Could you check a few things on this model? Use its own coordinates, in mm. A direction names the side the tool comes from. Round coordinates to 2 decimals unless told otherwise and drop trailing zeros. Write each loop counter-clockwise with the first axis right and the second up, starting at its lowest first coordinate (ties: lowest second). Pieces come first, ordered by that corner, then holes.
```python
from build123d import *

# Parameters (mm, degrees)
F0_R     = 9.525
F1_DEPTH = 12.7


with BuildPart() as f1:
    # F0 (on Top) → F1 (new body, symmetric)
    with BuildSketch(Plane.XY):
        with BuildLine():
            ThreePointArc((0, 38.1), (9.715033, 36.840577), (18.787791, 33.145571))
            Line((18.787791, 33.145571), (0, 50.8))
            Line((0, 50.8), (0, 38.1))
        make_face()
        with BuildLine():
            ThreePointArc((-20.773422, 31.938612), (-10.838983, 36.525696), (-0.010502, 38.099999))
            Line((-0.010502, 38.099999), (-25.138711, 43.864812))
            Line((-25.138711, 43.864812), (-20.773422, 31.938612))
        make_face()
        with BuildLine():
            ThreePointArc((-34.823787, 15.45684), (-28.994389, 24.717107), (-20.773422, 31.938612))
            Line((-20.773422, 31.938612), (-44.983609, 23.077076))
            Line((-44.983609, 23.077076), (-34.823787, 15.45684))
        make_face()
        with BuildLine():
            ThreePointArc((-37.621473, -6.019531), (-37.780783, 4.921632), (-34.823787, 15.45684))
            Line((-34.823787, 15.45684), (-50.292867, -5.1676))
            Line((-50.292867, -5.1676), (-37.621473, -6.019531))
        make_face()
        with BuildLine():
            Line((-39.350893, -31.74246), (-28.26246, -25.550799))
            ThreePointArc((-28.26246, -25.550799), (-34.358999, -16.46418), (-37.621473, -6.019531))
            Line((-37.621473, -6.019531), (-39.350893, -31.74246))
        make_face()
        with BuildLine():
            Line((-15.693389, -48.060318), (-9.770946, -36.825787))
            ThreePointArc((-9.770946, -36.825787), (-19.834726, -32.529889), (-28.26246, -25.550799))
            Line((-28.26246, -25.550799), (-15.693389, -48.060318))
        make_face()
        with BuildLine():
            Line((13.03515, -48.848346), (11.877897, -36.201182))
            ThreePointArc((11.877897, -36.201182), (1.098792, -38.084152), (-9.770946, -36.825787))
            Line((-9.770946, -36.825787), (13.03515, -48.848346))
        make_face()
        with BuildLine():
            Line((37.55164, -33.851957), (29.688458, -23.878975))
            ThreePointArc((29.688458, -23.878975), (21.677169, -31.332257), (11.877897, -36.201182))
            Line((11.877897, -36.201182), (37.55164, -33.851957))
        make_face()
        with BuildLine():
            Line((49.933612, -7.916716), (37.906115, -3.838811))
            ThreePointArc((37.906115, -3.838811), (35.251363, -14.455151), (29.688458, -23.878975))
            Line((29.688458, -23.878975), (49.933612, -7.916716))
        make_face()
        with BuildLine():
            ThreePointArc((33.881408, 17.425849), (37.030336, 8.964607), (38.1, 0))
            ThreePointArc((38.1, 0), (38.051498, -1.921852), (37.906115, -3.838811))
            Line((37.906115, -3.838811), (46.184261, 20.577008))
            Line((46.184261, 20.577008), (33.881408, 17.425849))
        make_face()
        with BuildLine():
            ThreePointArc((18.787791, 33.145571), (27.482514, 26.387903), (33.881408, 17.425849))
            Line((33.881408, 17.425849), (27.484554, 42.400641))
            Line((27.484554, 42.400641), (18.787791, 33.145571))
        make_face()
        with BuildLine():
            ThreePointArc((37.906115, -3.838811), (38.051498, -1.921852), (38.1, 0))
            ThreePointArc((38.1, 0), (37.030336, 8.964607), (33.881408, 17.425849))
            ThreePointArc((33.881408, 17.425849), (27.482514, 26.387903), (18.787791, 33.145571))
            ThreePointArc((18.787791, 33.145571), (9.715033, 36.840577), (0, 38.1))
            ThreePointArc((0, 38.1), (-0.005251, 38.1), (-0.010502, 38.099999))
            ThreePointArc((-0.010502, 38.099999), (-10.838983, 36.525696), (-20.773422, 31.938612))
            ThreePointArc((-20.773422, 31.938612), (-28.994389, 24.717107), (-34.823787, 15.45684))
            ThreePointArc((-34.823787, 15.45684), (-37.780783, 4.921632), (-37.621473, -6.019531))
            ThreePointArc((-37.621473, -6.019531), (-34.358999, -16.46418), (-28.26246, -25.550799))
            ThreePointArc((-28.26246, -25.550799), (-19.834726, -32.529889), (-9.770946, -36.825787))
            ThreePointArc((-9.770946, -36.825787), (1.098792, -38.084152), (11.877897, -36.201182))
            ThreePointArc((11.877897, -36.201182), (21.677169, -31.332257), (29.688458, -23.878975))
            ThreePointArc((29.688458, -23.878975), (35.251363, -14.455151), (37.906115, -3.838811))
        make_face()
        Circle(F0_R, mode=Mode.SUBTRACT)
    extrude(amount=F1_DEPTH, both=True)


solid = f1.part
```
Q1. If I drill on L1, parallel to X at y = -28.5, z = -4; L2, parallel to Y at x = 34.5, z = -5; L3, parallel to X at y = 6, z = 5, over which ranges is the centre line in solid material (lowest first)?
Q2. I'm going to push flat-ended pins straight in: pin 1 Ø4 at (y, z) = (27.5, 4.5) entering from +X; pin 2 Ø8 at (y, z) = (6.5, 9) entering from -X; pin 3 Ø12 at (y, z) = (39.5, 8.5) entering from +X. Where does each tip first touch, or does it pass through?
Q3. On a 3-axis mill with a long thin cutter (end or side, diameter ignored), from which of +Z, -Z, +X, -X, +Y, -Y can I reach the whole of each face in a straight line? I mean faces 1 (the flat face through (39.67, -16.01, 0.18)), 2 (the flat face through (-42.45, 5.29, 0.18)), 3 (the flat face through (-12.774, -42.522, 0.178)). Say none if no direction works.
Q4. We'd pull the mould along X, two halves only. Please class faces 4 (the flat face through (-22.99, 37.99, 0.18)), 5 (the flat face through (-33.9, -28.7, 0.2)), 6 (the flat face through (41.987, 8.198, 0.178)), 7 (the flat face through (9.525, 41.849, 0.178)): pulls with the +X half, pulls with the -X half, needs draft (parallel to the pull), parting line crosses it, or undercut.
Q5. Imagine slicing it at C-C, the plane y = 0. Write out the boundary of the cut face in (x, z) (3 decimals).
Q6. Imagine slicing it at D-D, the plane x = -33.5. Write out the boundary of the cut face in (y, z), then the cut area to 3 significant figures.
Q7. Imagine slicing it at B-B, the plane x = 4. Write out the boundary of the cut face in (y, z), then the cut area to 3 significant figures.
Results found:
1. L1: x = -39.13 to -33.54, -26.62 to 33.33
1. L2: y = -34.13 to -29.98, -20.09 to 17.58
1. L3: x = -41.92 to -7.4, 7.4 to 41.24
2. pin 1: stops at x = 31.81
2. pin 2: stops at x = -44.54
2. pin 3: stops at x = 29.76
3. face 1: +Z, -Z, +X
3. face 2: +Z, -Z, -X
3. face 3: +Z, -Z, -Y
4. face 4: pulls with the -X half
4. face 5: undercut
4. face 6: pulls with the +X half
4. face 7: undercut
5. outline: (-46.417, -12.7) - (-9.525, -12.7) - (-9.525, 12.7) - (-46.417, 12.7) - close; (9.525, -12.7) - (39.208, -12.7) - (39.208, 12.7) - (9.525, 12.7) - close
6. outline: (-28.48, -12.7) - (27.28, -12.7) - (27.28, 12.7) - (-28.48, 12.7) - close
6. area: 1,420 mm2
7. outline: (-44.09, -12.7) - (-8.64, -12.7) - (-8.64, 12.7) - (-44.09, 12.7) - close; (8.64, -12.7) - (47.04, -12.7) - (47.04, 12.7) - (8.64, 12.7) - close
7. area: 1,880 mm2
